```python
from build123d import *

# Parameters (mm, degrees)
SKETCH1_R           = 2.5
BOSS_EXTRUDE1_DEPTH = 189.096108091
SCALE_2_SCALE       = 3
SCALE_3_SCALE       = 6
SCALE_5_SCALE       = 2
SCALE_6_SCALE       = 0.25
SCALE_7_SCALE       = 0.125
SCALE_8_SCALE       = 0.25
SCALE_9_SCALE       = 4
SCALE_10_SCALE      = 4
OTHER_START         = 7.55
OTHER_1_OUTLINE_R   = 5
OTHER_1_DEPTH       = 10
SCALE_11_SCALE      = 0.111111111


# Read off the part's stored shape, not the designer's step: 孔1
with BuildPart() as part:
    # Sketch1 → Boss-Extrude1 (new body)
    with BuildSketch(Plane.XY):
        with BuildLine():
            Line((2.839339828, 3.9), (5.5, 6.560660172))
            Line((5.5, 6.560660172), (5.5, 8.2))
            Line((5.5, 8.2), (3.1, 8.2))
            Line((3.1, 8.2), (3.1, 9.5))
            Line((3.1, 9.5), (3.6, 9.5))
            Line((3.6, 9.5), (3.6, 10))
            Line((3.6, 10), (8.5, 10))
            ThreePointArc((8.5, 10), (9.560660172, 9.560660172), (10, 8.5))
            Line((10, 8.5), (10, 3.6))
            Line((10, 3.6), (9.5, 3.6))
            Line((9.5, 3.6), (9.5, 3.1))
            Line((9.5, 3.1), (8.2, 3.1))
            Line((8.2, 3.1), (8.2, 5.5))
            Line((8.2, 5.5), (6.560660172, 5.5))
            Line((6.560660172, 5.5), (3.9, 2.839339828))
            Line((3.9, 2.839339828), (3.9, -2.839339828))
            Line((3.9, -2.839339828), (6.560660172, -5.5))
            Line((6.560660172, -5.5), (8.2, -5.5))
            Line((8.2, -5.5), (8.2, -3.1))
            Line((8.2, -3.1), (9.5, -3.1))
            Line((9.5, -3.1), (9.5, -3.6))
            Line((9.5, -3.6), (10, -3.6))
            Line((10, -3.6), (10, -8.5))
            ThreePointArc((10, -8.5), (9.560660172, -9.560660172), (8.5, -10))
            Line((8.5, -10), (3.6, -10))
            Line((3.6, -10), (3.6, -9.5))
            Line((3.6, -9.5), (3.1, -9.5))
            Line((3.1, -9.5), (3.1, -8.2))
            Line((3.1, -8.2), (5.5, -8.2))
            Line((5.5, -8.2), (5.5, -6.560660172))
            Line((5.5, -6.560660172), (2.839339828, -3.9))
            Line((2.839339828, -3.9), (-2.839339828, -3.9))
            Line((-2.839339828, -3.9), (-5.5, -6.560660172))
            Line((-5.5, -6.560660172), (-5.5, -8.2))
            Line((-5.5, -8.2), (-3.1, -8.2))
            Line((-3.1, -8.2), (-3.1, -9.5))
            Line((-3.1, -9.5), (-3.6, -9.5))
            Line((-3.6, -9.5), (-3.6, -10))
            Line((-3.6, -10), (-8.5, -10))
            ThreePointArc((-8.5, -10), (-9.560660172, -9.560660172), (-10, -8.5))
            Line((-10, -8.5), (-10, -3.6))
            Line((-10, -3.6), (-9.5, -3.6))
            Line((-9.5, -3.6), (-9.5, -3.1))
            Line((-9.5, -3.1), (-8.2, -3.1))
            Line((-8.2, -3.1), (-8.2, -5.5))
            Line((-8.2, -5.5), (-6.560660172, -5.5))
            Line((-6.560660172, -5.5), (-3.9, -2.839339828))
            Line((-3.9, -2.839339828), (-3.9, 2.839339828))
            Line((-3.9, 2.839339828), (-6.560660172, 5.5))
            Line((-6.560660172, 5.5), (-8.2, 5.5))
            Line((-8.2, 5.5), (-8.2, 3.1))
            Line((-8.2, 3.1), (-9.5, 3.1))
            Line((-9.5, 3.1), (-9.5, 3.6))
            Line((-9.5, 3.6), (-10, 3.6))
            Line((-10, 3.6), (-10, 8.5))
            ThreePointArc((-10, 8.5), (-9.560660172, 9.560660172), (-8.5, 10))
            Line((-8.5, 10), (-3.6, 10))
            Line((-3.6, 10), (-3.6, 9.5))
            Line((-3.6, 9.5), (-3.1, 9.5))
            Line((-3.1, 9.5), (-3.1, 8.2))
            Line((-3.1, 8.2), (-5.5, 8.2))
            Line((-5.5, 8.2), (-5.5, 6.560660172))
            Line((-5.5, 6.560660172), (-2.839339828, 3.9))
            Line((-2.839339828, 3.9), (2.839339828, 3.9))
        make_face()
        with Locations((0, 0.235847297)):
            Circle(SKETCH1_R, mode=Mode.SUBTRACT)
    extrude(amount=BOSS_EXTRUDE1_DEPTH)


with BuildPart() as part_1:
    # 缩放比例2: scaled about (0, -0.027095247, 94.548054046)
    add(part.part.scale(SCALE_2_SCALE).moved(Location((0, 0.054190494, -189.096108092))))


with BuildPart() as part_2:
    # 缩放比例3: scaled about (0, -0.027095247, 94.548054045)
    add(part_1.part.scale(SCALE_3_SCALE).moved(Location((0, 0.135476235, -472.740270225))))


with BuildPart() as part_3:
    # 缩放比例5: scaled about (0, -0.027095249, 94.548054043)
    add(part_2.part.scale(SCALE_5_SCALE).moved(Location((0, 0.027095249, -94.548054043))))


with BuildPart() as part_4:
    # 缩放比例6: scaled about (0, -0.027095249, 94.548054044)
    add(part_3.part.scale(SCALE_6_SCALE).moved(Location((0, -0.020321437, 70.911040533))))


with BuildPart() as part_5:
    # 缩放比例7: scaled about (0, -0.027095249, 94.548054044)
    add(part_4.part.scale(SCALE_7_SCALE).moved(Location((0, -0.023708343, 82.729547289))))


with BuildPart() as part_6:
    # 缩放比例8: scaled about (0, -0.027095249, 94.548054044)
    add(part_5.part.scale(SCALE_8_SCALE).moved(Location((0, -0.020321437, 70.911040533))))


with BuildPart() as part_7:
    # 缩放比例9: scaled about (0, -0.027095249, 94.548054044)
    add(part_6.part.scale(SCALE_9_SCALE).moved(Location((0, 0.081285747, -283.644162132))))


with BuildPart() as part_8:
    # 缩放比例10: scaled about (0, -0.027095249, 94.548054044)
    add(part_7.part.scale(SCALE_10_SCALE).moved(Location((0, 0.081285747, -283.644162132))))

    # 孔1 outline → 孔1 (cut)
    with BuildSketch(Plane.YZ.offset(OTHER_START)):
        with Locations((7.344832291, -26.42806198)):
            Circle(OTHER_1_OUTLINE_R)
    extrude(amount=OTHER_1_DEPTH, mode=Mode.SUBTRACT)


with BuildPart() as part_9:
    # 缩放比例11: scaled about (-0.002946752, -0.028813034, 94.574865823)
    add(part_8.part.scale(SCALE_11_SCALE).moved(Location((-0.002619335, -0.025611586, 84.066547398))))


solid = part_9.part
```
Here's how the part is built. I have some questions about the finished solid (model axes, mm). A direction names the side the tool comes from. Coordinates: 2 decimals unless noted, no trailing zeros. One line per question, with ' | ' between items. Start each with the question number.
1. If we mould it in two halves opening along Y, with no side actions, what happens to faces 4 (the flat face through (-5.003, 3, 94)), 5 (the cylindrical face through (-1.25, 0.16, 93.91)), 6 (the flat face through (-3, 4.985, 94))? For each: released by +Y, released by -Y, zero draft, split by the parting line, or undercut.
2. Which directions (+Z, -Z, +X, -X, +Y, -Y) give clear straight access to the entire face, cutting with the end or side of a thin tool? Please do faces 1 (the flat face through (1.947, 0, 94)), 2 (the flat face through (0, 1.935, 94)), 3 (the flat face through (0, -1.965, 94)).
3. Please list where these lines run through material, in increasing order: line 1 along Y through (x, z) = (-3.5, 67); line 2 along Y through (x, z) = (2.25, 113.5); line 3 along X through (y, z) = (2.5, 112.5). Write a range as [from, to].
Model answer:
1) face 4: zero draft | face 5: undercut | face 6: released by +Y
2) face 1: +Z, -Z, +X | face 2: +Z, -Z, +Y | face 3: +Z, -Z, -Y
3) line 1: y = [-5.02, -2.77], [2.73, 4.98] | line 2: y = [-5.02, -4.12], [-2.8, -1.74], [1.71, 2.77], [4.08, 4.98] | line 3: x = [-5, -4.1], [-3.05, -1.99], [1.98, 3.04], [4.1, 5]
